from build123d import *

# Parameters (mm, degrees)
SKETCH_R           = 8
PAD_DEPTH          = 16
SKETCH001_W        = 1.89
SKETCH001_H        = 7.4
SKETCH002_R        = 2.5
POCKET_DEPTH       = 16.001
POCKET001_DEPTH    = 7.5
POLARPATTERN_COUNT = 20


with BuildPart() as part:
    # Sketch → Pad (new body)
    with BuildSketch(Plane.XY):
        Circle(SKETCH_R)
    extrude(amount=PAD_DEPTH)

    # Sketch001 → Groove (revolve, cut)
    with BuildSketch(Plane.XZ):
        with Locations((7.055, 10.8)):
            Rectangle(SKETCH001_W, SKETCH001_H)
    revolve(axis=Axis((0, 0, 0), (0, 0, 1)), mode=Mode.SUBTRACT)

    # Sketch002 (on Face7 of Groove) → Pocket (cut, through all)
    with BuildSketch(Plane.XY.offset(16)):
        Circle(SKETCH002_R)
    extrude(amount=-POCKET_DEPTH, mode=Mode.SUBTRACT)

    # Sketch003 (on Face3 of Pocket) → Pocket001 (cut)
    with BuildSketch(Plane.XY.offset(7.1)):
        with BuildLine():
            ThreePointArc((6.089542, 0.499581), (5.61, 0), (6.089542, -0.499581))
            ThreePointArc((6.089542, -0.499581), (6.11, 0), (6.089542, 0.499581))
        make_face()
    pocket001 = extrude(amount=POCKET001_DEPTH, mode=Mode.SUBTRACT)

    # PolarPattern: Pocket001 ×20 about axis
    polarpattern_axis = Axis((0, 0, 7.1), (0, 0, 1))
    for i in range(1, POLARPATTERN_COUNT):
        add(pocket001.rotate(polarpattern_axis, i * 360 / POLARPATTERN_COUNT), mode=Mode.SUBTRACT)


solid = part.part
Design review of the part built by this model. Coordinates are the model's own, in mm. A direction names the side the tool comes from. Give positions to 0.01 mm unless a question says otherwise; leave off trailing zeros. Loops run counter-clockwise (first coordinate to the right, second up) from the corner with the lowest first, then second, coordinate; pieces in that order, holes last. Notation, with made-up numbers: M 18,39 L 59,39 A19 cw 59,73 Z; hole C 8.25,74.5 d7. An arc over 180 degrees is marked long. Answer as a JSON object with one key per item and string values.
Item 1: We need section D-D (y = 2.75). State the section outline as (x, z) points.
Output values:
{"outline": "M -7.51,0 L 7.51,0 L 7.51,7.1 L 5.46,7.1 L 5.46,14.5 L 7.51,14.5 L 7.51,16 L -7.51,16 L -7.51,14.5 L -5.46,14.5 L -5.46,7.1 L -7.51,7.1 Z"}
Item 2: We need section A-A (y = 0). State the section outline as (x, z) points.
Output values:
{"outline": "M -8,0 L -2.5,0 L -2.5,16 L -8,16 L -8,14.5 L -6.11,14.5 L -6.11,14.6 L -5.61,14.6 L -5.61,7.1 L -8,7.1 Z; M 2.5,0 L 8,0 L 8,7.1 L 5.61,7.1 L 5.61,14.6 L 6.11,14.6 L 6.11,14.5 L 8,14.5 L 8,16 L 2.5,16 Z"}
Item 3: For P1, Ø1.5, axis at y = -1, z = 4.5, coming from the +X side; P2, Ø2, axis at x = 0, z = 13, coming from the -Y side; P3, Ø3, axis at y = -5.5, z = 4.5, coming from the -X side, all flat-tipped, find the tip position at first contact; note any pin that passes through.
Output values:
{"P1": "stops at x = 8", "P2": "stops at y = -6.09", "P3": "stops at x = -6.93"}
Item 4: Mouldability with a two-part tool opening along Y and no side actions: class faces 5 (the face through (-6.034, 0.962, 10.852)), 6 (the face through (2, 2, 16)), 7 (the face through (-1.72, -5.34, 10.8)) as pulls with the +Y half, pulls with the -Y half, needs draft (parallel to the pull), parting line crosses it, or undercut.
Output values:
{"face 5": "pulls with the +Y half", "face 6": "needs draft", "face 7": "undercut"}
Item 5: We need section C-C (z = 6.5). State the section outline as (x, y) points.
Output values:
{"outline": "C 0,0 d16; hole C 0,0 d5"}
Item 6: Wall thickness on line 1 along Z through (x, y) = (7.25, 2); line 2 along Y through (x, z) = (0, 5.5); line 3 along X through (y, z) = (-5.5, 12): over which ranges is each line inside the solid? List them lowest first.
Output values:
{"line 1": "z = 0 to 7.1, 14.5 to 16", "line 2": "y = -8 to -2.5, 2.5 to 8", "line 3": "x = -2.66 to -2.28, -1.5 to 1.5, 2.28 to 2.66"}
Item 7: Machinability: for faces 1 (the face through (4.545, -3.289, 10.798)), 2 (the face through (-0.962, -6.034, 10.852)), 3 (the face through (6.034, -0.962, 10.852)), 4 (the face through (2.78, 5.44, 10.85)), which of the approach directions +Z, -Z, +X, -X, +Y, -Y give a long, thin tool a straight path to every point of the face, cutting with its end or side? Answer none if there is none.
Output values:
{"face 1": "none", "face 2": "-X, -Y", "face 3": "+X, -Y", "face 4": "+X, +Y"}
